from build123d import *

# Parameters (mm, degrees)
SKETCH1_W           = 29.3
SKETCH1_H           = 3.44
BOSS_EXTRUDE1_DEPTH = 120
FILLET1_R           = 0.75
CUT_EXTRUDE1_REACH  = 8.76
SKETCH2_R           = 1.45


with BuildPart() as part:
    # Sketch1 → Boss-Extrude1 (new body)
    with BuildSketch(Plane(origin=(0, 0, 0), x_dir=(0, 0, -1), z_dir=(1, 0, 0))):
        Polygon((-16.25, 0), (-16.25, 5.1), (-35, 5.1), (-35, 6.76), (35, 6.76), (35, 5.1), (16.25, 5.1), (16.25, 0), align=None)
        with Locations((0, 3.38)):
            Rectangle(SKETCH1_W, SKETCH1_H, mode=Mode.SUBTRACT)
    extrude(amount=BOSS_EXTRUDE1_DEPTH)

    # Fillet1
    fillet1_edges = [part.edges().sort_by_distance(p)[0] for p in [
        (60, 0, 16.25),
        (60, 5.1, 35),
        (60, 6.76, 35),
        (60, 6.76, -35),
        (60, 5.1, -35),
        (60, 0, -16.25),
    ]]
    fillet(fillet1_edges, radius=FILLET1_R)

    # Sketch2 → Cut-Extrude1 (cut, up to next)
    with BuildSketch(Plane(origin=(0, 6.76, 0), x_dir=(1, 0, 0), z_dir=(0, 1, 0)), mode=Mode.PRIVATE) as cut_extrude1_sk1:
        with Locations((115, 30)):
            Circle(SKETCH2_R)
    cut_extrude1_tool1 = extrude(cut_extrude1_sk1.sketch, amount=-CUT_EXTRUDE1_REACH, mode=Mode.PRIVATE) & part.part
    add(cut_extrude1_tool1.solids().sort_by_distance((115, 6.76, -30))[0], mode=Mode.SUBTRACT)
    # Sketch2 → Cut-Extrude1 (cut, up to next)
    with BuildSketch(Plane(origin=(0, 6.76, 0), x_dir=(1, 0, 0), z_dir=(0, 1, 0)), mode=Mode.PRIVATE) as cut_extrude1_sk2:
        with Locations((5, 30)):
            Circle(SKETCH2_R)
    cut_extrude1_tool2 = extrude(cut_extrude1_sk2.sketch, amount=-CUT_EXTRUDE1_REACH, mode=Mode.PRIVATE) & part.part
    add(cut_extrude1_tool2.solids().sort_by_distance((5, 6.76, -30))[0], mode=Mode.SUBTRACT)
    # Sketch2 → Cut-Extrude1 (cut, up to next)
    with BuildSketch(Plane(origin=(0, 6.76, 0), x_dir=(1, 0, 0), z_dir=(0, 1, 0)), mode=Mode.PRIVATE) as cut_extrude1_sk3:
        with Locations((5, -30)):
            Circle(SKETCH2_R)
    cut_extrude1_tool3 = extrude(cut_extrude1_sk3.sketch, amount=-CUT_EXTRUDE1_REACH, mode=Mode.PRIVATE) & part.part
    add(cut_extrude1_tool3.solids().sort_by_distance((5, 6.76, 30))[0], mode=Mode.SUBTRACT)
    # Sketch2 → Cut-Extrude1 (cut, up to next)
    with BuildSketch(Plane(origin=(0, 6.76, 0), x_dir=(1, 0, 0), z_dir=(0, 1, 0)), mode=Mode.PRIVATE) as cut_extrude1_sk4:
        with Locations((115, -30)):
            Circle(SKETCH2_R)
    cut_extrude1_tool4 = extrude(cut_extrude1_sk4.sketch, amount=-CUT_EXTRUDE1_REACH, mode=Mode.PRIVATE) & part.part
    add(cut_extrude1_tool4.solids().sort_by_distance((115, 6.76, 30))[0], mode=Mode.SUBTRACT)


solid = part.part
CAD build for the part. Positions are in the model's coordinates, mm. A direction names the side the tool comes from. Coordinates: 2 decimals unless noted, no trailing zeros. Order: outer loops, then holes, each group sorted by start corner. A loop starts at its lowest first (then second) coordinate and runs counter-clockwise, first axis right, second up.
Item 1: Two-plate mould, pull along Z, no slides. Class faces 1 (the face through (59, 0, 0)), 2 (the face through (59, 3, 16.25)), 3 (the face through (59, 1.66, 0)), 4 (the face through (59, 5.1, 0)): +Z half, -Z half, draft (parallel to the pull), parting line (faces both ways), or undercut.
Check sheet entries:
face 1: draft
face 2: +Z half
face 3: undercut
face 4: undercut
Item 2: Band-saw the part on A-A on z = 30. List the corners of the cut face in (x, y), plus the area to 3 significant figures.
Check sheet entries:
outline: (0, 5.1) - (3.55, 5.1) - (3.55, 6.76) - (0, 6.76) - close; (6.45, 5.1) - (113.55, 5.1) - (113.55, 6.76) - (6.45, 6.76) - close; (116.45, 5.1) - (120, 5.1) - (120, 6.76) - (116.45, 6.76) - close
area: 190 mm2
Item 3: Band-saw the part on D-D on x = 33. List the corners of the cut face in (y, z), plus the area to 3 significant figures.
Check sheet entries:
outline: (0, -15.5) arc R0.75 ccw to (0.75, -16.25) - (5.1, -16.25) - (5.1, -34.25) arc R0.75 ccw to (5.85, -35) - (6.01, -35) arc R0.75 ccw to (6.76, -34.25) - (6.76, 34.25) arc R0.75 ccw to (6.01, 35) - (5.85, 35) arc R0.75 ccw to (5.1, 34.25) - (5.1, 16.25) - (0.75, 16.25) arc R0.75 ccw to (0, 15.5) - close; hole (1.66, -14.65) - (5.1, -14.65) - (5.1, 14.65) - (1.66, 14.65) - close
area: 180 mm2
Item 4: Drill centre lines: L1, parallel to Z at x = 5, y = 5.65; L2, parallel to X at y = 5.5, z = 30; L3, parallel to Z at x = 17.5, y = 3.5. Where is each one in solid material? Low to high.
Check sheet entries:
L1: z = -34.97 to -31.45, -28.55 to 28.55, 31.45 to 34.97
L2: x = 0 to 3.55, 6.45 to 113.55, 116.45 to 120
L3: z = -16.25 to -14.65, 14.65 to 16.25
Item 5: Pin check, flat tips, straight feed: pin 1 Ø2 at (x, y) = (72.5, 4) entering from -Z; pin 2 Ø1.5 at (x, y) = (77, 4) entering from +Z; pin 3 Ø9 at (x, z) = (75, -28) entering from -Y. Stop position of each tip, or through.
Check sheet entries:
pin 1: stops at z = -16.25
pin 2: stops at z = 16.25
pin 3: stops at y = 5.1
Item 6: Band-saw the part on B-B on x = 5. List the corners of the cut face in (y, z), plus the area to 3 significant figures.
Check sheet entries:
outline: (0, -15.5) arc R0.75 ccw to (0.75, -16.25) - (5.1, -16.25) - (5.1, -28.55) - (6.76, -28.55) - (6.76, 28.55) - (5.1, 28.55) - (5.1, 16.25) - (0.75, 16.25) arc R0.75 ccw to (0, 15.5) - close; (5.1, -34.25) arc R0.75 ccw to (5.85, -35) - (6.01, -35) arc R0.75 ccw to (6.76, -34.25) - (6.76, -31.45) - (5.1, -31.45) - close; (5.1, 31.45) - (6.76, 31.45) - (6.76, 34.25) arc R0.75 ccw to (6.01, 35) - (5.85, 35) arc R0.75 ccw to (5.1, 34.25) - close; hole (1.66, -14.65) - (5.1, -14.65) - (5.1, 14.65) - (1.66, 14.65) - close
area: 171 mm2
Item 7: 3-axis set-ups, long thin cutter, end or side, ignore diameter. For faces 5 (the face through (59, 5.1, 25)), 6 (the face through (59, 3, -14.65)), 7 (the face through (59, 6.76, 0)), 8 (the face through (59, 3, -16.25)): which of +Z, -Z, +X, -X, +Y, -Y reach the whole face in a straight line?
Check sheet entries:
face 5: +Z, +X, -X, -Y
face 6: +X, -X
face 7: +Z, -Z, +X, -X, +Y
face 8: -Z, +X, -X, -Y
Item 8: Band-saw the part on C-C on z = 9. List the corners of the cut face in (x, y), plus the area to 3 significant figures.
Check sheet entries:
outline: (0, 0) - (120, 0) - (120, 1.66) - (0, 1.66) - close; (0, 5.1) - (120, 5.1) - (120, 6.76) - (0, 6.76) - close
area: 398 mm2
